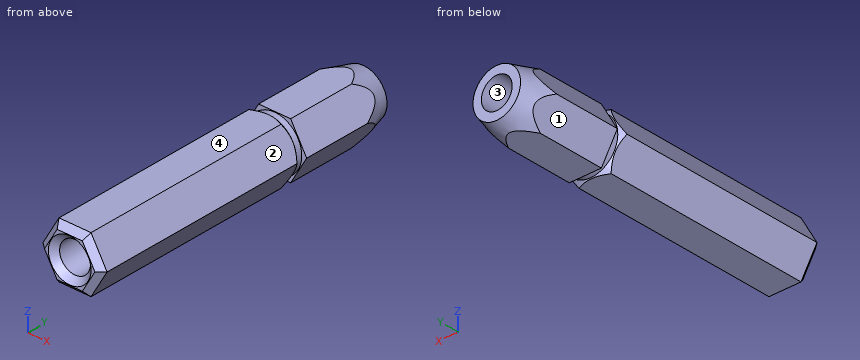
```python
from build123d import *

# Parameters (mm, degrees)
EXTRUDE1_DEPTH     = 84.1375
SKETCH4_R          = 3.96875
CUT_EXTRUDE1_DEPTH = 85.842184608
CHAMFER1_SIZE      = 1.524


with BuildPart() as part:
    # Sketch1 → Extrude1 (new body)
    with BuildSketch(Plane(origin=(0, 0, 0), x_dir=(1, 0, 0), z_dir=(0, 1, 0))):
        Polygon((4.124445986, -7.14375), (8.248891971, 0), (4.124445986, 7.14375), (-4.124445986, 7.14375), (-8.248891971, 0), (-4.124445986, -7.14375), align=None)
    extrude(amount=EXTRUDE1_DEPTH)

    # Sketch4 → Cut-Extrude1 (cut, through all)
    with BuildSketch(Plane(origin=(0, 84.1375, 0), x_dir=(-1, 0, 0), z_dir=(0, 1, 0))):
        with Locations(Location((0, 0, 0), (0, 0, 90))):
            Circle(SKETCH4_R)
    extrude(amount=-CUT_EXTRUDE1_DEPTH, mode=Mode.SUBTRACT)

    # Sketch2 → Cut-Revolve1 (revolve, cut)
    with BuildSketch(Plane(origin=(0, 0, 0), x_dir=(-0.500000000000001, 0, -0.866025403784438), z_dir=(0.866025403784438, 0, -0.500000000000001)), mode=Mode.PRIVATE) as cut_revolve1_sk:
        Polygon((8.248891971, 84.1375), (8.248891971, 76.2), (6.122045256, 84.1375), align=None)
    revolve(cut_revolve1_sk.sketch.rotate(Axis((0, -6.288333001, 0), (0, 1, 0)), 330), axis=Axis((0, -6.288333001, 0), (0, 1, 0)), mode=Mode.SUBTRACT)

    # Sketch3 → Cut-Revolve2 (revolve, cut)
    with BuildSketch(Plane(origin=(0, 0, 0), x_dir=(-0.500000000000001, 0, -0.866025403784438), z_dir=(0.866025403784438, 0, -0.500000000000001)), mode=Mode.PRIVATE) as cut_revolve2_sk:
        Polygon((8.248891971, 55.949608029), (6.985, 57.2135), (6.985, 58.7375), (8.248891971, 58.7375), align=None)
    revolve(cut_revolve2_sk.sketch.rotate(Axis((0, -5.572817584, 0), (0, 1, 0)), 330), axis=Axis((0, -5.572817584, 0), (0, 1, 0)), mode=Mode.SUBTRACT)

    # Chamfer1
    chamfer1_edges = [part.edges().sort_by_distance(p)[0] for p in [
        (0, 0, -3.96875),
        (-6.186668978, 0, 3.571875),
        (-6.186668978, 0, -3.571875),
        (0, 0, -7.14375),
        (6.186668978, 0, -3.571875),
        (6.186668978, 0, 3.571875),
        (0, 0, 7.14375),
    ]]
    chamfer(chamfer1_edges, length=CHAMFER1_SIZE)


solid = part.part
```
Geometry: final body of the model. Coordinates: model frame, mm. Face numbers are marked on the shaded views. Coordinates: 2 decimals unless noted, no trailing zeros. Loops run counter-clockwise (first coordinate to the right, second up) from the corner with the lowest first, then second, coordinate; pieces in that order, holes last. Notation, with made-up numbers: (16.25, -38) -> (59.25, -38) arc R17 ccw to (59.25, -10) -> close; hole circle Ø10 at (80.25, 57.25). An arc over 180 degrees is marked (long way). Use a Markdown table: item, result. Add a question column.
(1) Section query C-C, the plane y = 78.5. Return loops of the section in (x, z).
(2) Line query: line 1 along Z through (x, y) = (-3.5, 21); line 2 along Z through (x, y) = (2, 41); line 3 along X through (y, z) = (9.5, -3.5). Output: solid intervals per line, ascending.
(3) Mould query, pull axis X, two halves, no side actions, for the marked faces 1, 2, 3 and 4. Classes: pulls with the +X half, pulls with the -X half, needs draft (parallel to the pull), parting line crosses it, or undercut.
(4) Pin query (flat end, axial travel): pin 1 Ø1.5 at (y, z) = (11, -4.5) entering from +X; pin 2 Ø1.5 at (y, z) = (58, -4) entering from +X; pin 3 Ø5 at (x, z) = (0, 0) entering from +Y; pin 4 Ø6 at (x, y) = (5.5, 73.5) entering from +Z. Return the tip coordinate at first contact, or that it passes through.
(5) Section query B-B, the plane y = 62.5. Return loops of the section in (x, z), plus the area to 3 significant figures.
Answer:
| question | item | result |
|---|---|---|
| 1 | outline | (-7.53, -1.24) -> (-4.84, -5.9) arc R7.63 ccw to (-2.69, -7.14) -> (2.69, -7.14) arc R7.63 ccw to (4.84, -5.9) -> (7.53, -1.24) arc R7.63 ccw to (7.53, 1.24) -> (4.84, 5.9) arc R7.63 ccw to (2.69, 7.14) -> (-2.69, 7.14) arc R7.63 ccw to (-4.84, 5.9) -> (-7.53, 1.24) arc R7.63 ccw to start; hole circle Ø7.94 at (0, 0) |
| 2 | line 1 | z = -7.14 to -1.87, 1.87 to 7.14 |
| 2 | line 2 | z = -7.14 to -3.43, 3.43 to 7.14 |
| 2 | line 3 | x = -6.23 to -1.87, 1.87 to 6.23 |
| 3 | face 1 | pulls with the -X half |
| 3 | face 2 | pulls with the +X half |
| 3 | face 3 | undercut |
| 3 | face 4 | needs draft |
| 4 | pin 1 | stops at x = 6.08 |
| 4 | pin 2 | stops at x = 6.18 |
| 4 | pin 3 | passes through |
| 4 | pin 4 | stops at z = 7.14 |
| 5 | outline | (-8.25, 0) -> (-4.12, -7.14) -> (4.12, -7.14) -> (8.25, 0) -> (4.12, 7.14) -> (-4.12, 7.14) -> close; hole circle Ø7.94 at (0, 0) |
| 5 | area | 127 mm^2 |
